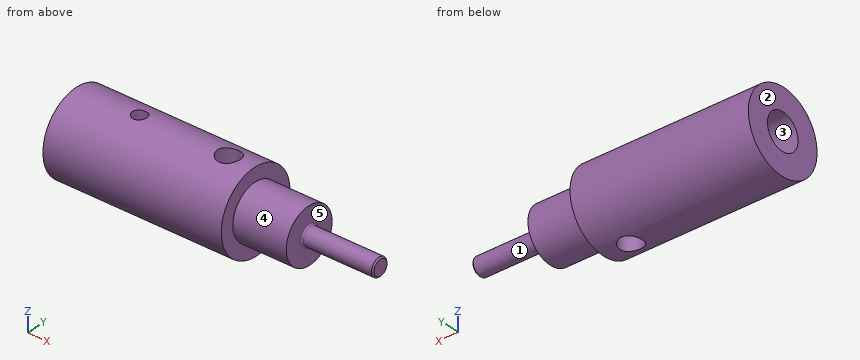
from build123d import *

# Parameters (mm, degrees)
FASE1_SIZE                           = 0.15
SKIZZE5_W                            = 0.8
SKIZZE5_H                            = 4.5
SKIZZE7_R                            = 1.25
SCHNITT_LINEAR_AUSTRAGEN2_DEPTH      = 5.50000011
SCHNITT_LINEAR_AUSTRAGEN2_DEPTH_BACK = 5.5000001
VERRUNDUNG1_R                        = 0.2


with BuildPart() as part:
    # Skizze1 → Rotation1 (revolve)
    with BuildSketch(Plane.XY):
        Polygon((0, 4.5), (0, 2), (14, 2), (15.201721238, 0), (34, 0), (34, 1), (26, 1), (26, 3), (20, 3), (20, 4.5), align=None)
    revolve(axis=Axis((0, 0, 0), (1, 0, 0)))

    # Fase1
    fase1_edges = [part.edges().sort_by_distance(p)[0] for p in [
        (34, -1, 0),
    ]]
    chamfer(fase1_edges, length=FASE1_SIZE)

    # Skizze5 → M2 Gewindebohrung1 (revolve, cut)
    with BuildSketch(Plane.YZ.offset(7)):
        with Locations((0.4, 2.25)):
            Rectangle(SKIZZE5_W, SKIZZE5_H)
    revolve(axis=Axis((7, 0, -6.35), (0, 0, 1)), mode=Mode.SUBTRACT)

    # Skizze7 → Schnitt-Linear austragen2 (cut, two sides)
    with BuildSketch(Plane.XY) as schnitt_linear_austragen2_sk:
        with Locations((17, 0)):
            Circle(SKIZZE7_R)
    extrude(amount=SCHNITT_LINEAR_AUSTRAGEN2_DEPTH, mode=Mode.SUBTRACT)
    extrude(schnitt_linear_austragen2_sk.sketch, amount=-SCHNITT_LINEAR_AUSTRAGEN2_DEPTH_BACK, mode=Mode.SUBTRACT)

    # Verrundung1
    verrundung1_edges = [part.edges().sort_by_distance(p)[0] for p in [
        (26, -1, 0),
    ]]
    fillet(verrundung1_edges, radius=VERRUNDUNG1_R)


solid = part.part
Read the model definition and answer for the solid it produces. Units are mm, in the model's axes. Face numbers are marked on the shaded views. A direction names the side the tool comes from. Give positions to 0.01 mm unless a question says otherwise; leave off trailing zeros. Loops run counter-clockwise (first coordinate to the right, second up) from the corner with the lowest first, then second, coordinate; pieces in that order, holes last. Notation, with made-up numbers: (-6, 19.5) - (22, 19.5) arc R26 cw to (22, 48.5) - close; hole circle Ø10 at (-25.5, -0.5). An arc over 180 degrees is marked (long way). Answer as CSV lines item,"result". Start each with the question number.
1) Find section C-C (x = 19.5). Write down the section's boundary in (y, z), then the cut area to 3 significant figures.
2) Find section B-B (x = 5). Write down the section's boundary in (y, z).
3) Each of these flat-tipped pins is pushed along its axis until it touches: pin 1 Ø1 at (y, z) = (0, 2) entering from +X; pin 2 Ø1.5 at (x, y) = (23, 0.5) entering from +Z. Where does it stop, or does it pass through?
4) Straight lines are drawn through the part: L1, parallel to X at y = 0, z = 3.1; L2, parallel to X at y = -0.5, z = 2.5; L3, parallel to X at y = 0, z = -2.35. For each, find the intervals that lie inside material, in ascending order. Write a range as from..to.
5) Which of the six approach directions +Z, -Z, +X, -X, +Y, -Y give full straight-line access (tool end or side, diameter ignored) to the marked faces 1 and 2?
6) Determine the mould class of the marked faces 3, 4 and 5 for opening direction Y: released by +Y, released by -Y, zero draft, split by the parting line, or undercut.
7) Find section A-A (z = 3.5). Write down the section's boundary in (x, y).
Findings below:
1,outline,"circle Ø9 at (0, 0)"
1,area,"63.6 mm^2"
2,outline,"circle Ø9 at (0, 0); hole circle Ø4 at (0, 0)"
3,pin 1,"x = 26"
3,pin 2,"z = 3"
4,L1,"0..6.2, 7.8..15.75, 18.25..20"
4,L2,"0..6.38, 7.62..15.85, 18.15..26"
4,L3,"0..15.75, 18.25..26"
5,face 1,"+X"
5,face 2,"+Z, -Z, -X, +Y, -Y"
6,face 3,"undercut"
6,face 4,"split by the parting line"
6,face 5,"zero draft"
7,outline,"(0, -2.83) - (20, -2.83) - (20, 2.83) - (0, 2.83) - close; hole circle Ø1.6 at (7, 0); hole circle Ø2.5 at (17, 0)"
